Answer from the drawing. Dimensions are ordinates in mm from the lowest x, y and z of the part. A direction names the side the tool comes from. Round coordinates to 2 decimals unless told otherwise and drop trailing zeros. Loops run counter-clockwise (first coordinate to the right, second up) from the corner with the lowest first, then second, coordinate; pieces in that order, holes last. Notation, with made-up numbers: (23.25, 4) - (53.25, 4) arc R23 ccw to (53.25, 21) - close; hole circle Ø7 at (89.5, 49). An arc over 180 degrees is marked (long way). Write item = value, one per line. Start each with the question number.
1) Section B-B, the plane z = 3.5 is taken. Determine the outline of the cut face in (x, y).
2) Section C-C, the plane y = 21 is taken. Determine the outline of the cut face in (x, z), and give its area (3 significant figures).
3) Straight lines are drawn through the part: line 1 along X through (y, z) = (27, 13); line 2 along X through (y, z) = (39, 11); line 3 along X through (y, z) = (48, 8). For each, find the intervals that lie inside material, in ascending order.
4) Section D-D, the plane z = 16 is taken. Determine the outline of the cut face in (x, y), and give its area (3 significant figures).
5) Given pin 1 Ø16 at (x, y) = (8, 18.5) entering from -Z; pin 2 Ø9.5 at (y, z) = (19.5, 4) entering from -X; pin 3 Ø5 at (y, z) = (37.5, 4) entering from +X, each flat-ended and moving along its own axis, determine where each tip first touches the part or whether it passes through.
6) A tool of negligible diameter and unlimited length cuts with its end or side. For the marked faces 1, 2 and 3, from which of +Z, -Z, +X, -X, +Y, -Y can it reach the whole face along a straight path? Write none if from no direction.
7) Section A-A, the plane y = 32 is taken. Determine the outline of the cut face in (x, z), and give its area (3 significant figures).
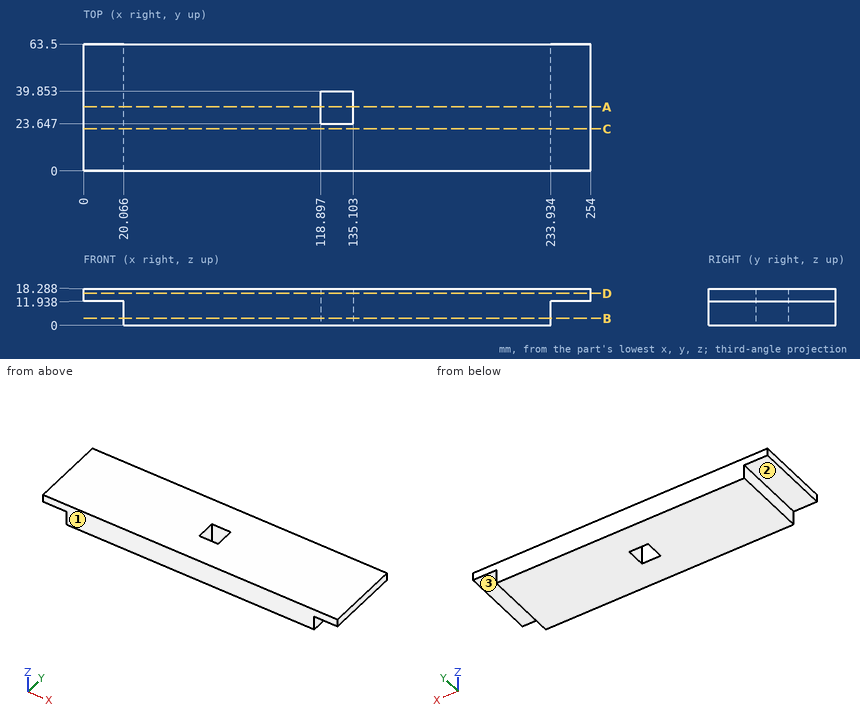
Geometry check:
q1.outline = (20.07, 0) - (233.93, 0) - (233.93, 63.5) - (20.07, 63.5) - close; hole (118.9, 23.65) - (135.1, 23.65) - (135.1, 39.85) - (118.9, 39.85) - close
q2.outline = (0, 11.94) - (20.07, 11.94) - (20.07, 0) - (233.93, 0) - (233.93, 11.94) - (254, 11.94) - (254, 18.29) - (0, 18.29) - close
q2.area = 4,170 mm2
q3.line_1 = 0 to 118.9, 135.1 to 254
q3.line_2 = 20.07 to 118.9, 135.1 to 233.93
q3.line_3 = 20.07 to 233.93
q4.outline = (0, 0) - (254, 0) - (254, 63.5) - (0, 63.5) - close; hole (118.9, 23.65) - (135.1, 23.65) - (135.1, 39.85) - (118.9, 39.85) - close
q4.area = 15,900 mm2
q5.pin_1 = 11.94
q5.pin_2 = 20.07
q5.pin_3 = 233.93
q6.face_1 = +Z, -Z, +X, -X, -Y
q6.face_2 = -Z, -X, +Y, -Y
q6.face_3 = -Z, +X, +Y, -Y
q7.outline = (0, 11.94) - (20.07, 11.94) - (20.07, 0) - (118.9, 0) - (118.9, 18.29) - (0, 18.29) - close; (135.1, 0) - (233.93, 0) - (233.93, 11.94) - (254, 11.94) - (254, 18.29) - (135.1, 18.29) - close
q7.area = 3,870 mm2
